Geometry check sheet. Reference: the model listing, model coordinates, mm. A direction names the side the tool comes from. Give positions to 0.01 mm unless a question says otherwise; leave off trailing zeros. Order: outer loops, then holes, each group sorted by start corner. A loop starts at its lowest first (then second) coordinate and runs counter-clockwise, first axis right, second up. Notation, with made-up numbers: M 88,14.5 L 125,14.5 A21 ccw 125,35.5 Z; hole C 5.25,2.5 d4. An arc over 180 degrees is marked long. Answer as CSV lines item,"result".
Autodesk Inventor part; units mm, degrees
ref_plane "YZ Plane" through (0, 0, 0) normal (1, 0, 0) x (0, 1, 0)
ref_plane "XZ Plane" through (0, 0, 0) normal (0, 1, 0) x (-1, 0, 0)
ref_plane "XY Plane" through (0, 0, 0) normal (0, 0, 1) x (1, 0, 0)
sketch "Sketch1" plane through (0, 0, 0) normal (0, 0, 1) x (1, 0, 0)
  line L0 (0, 0) -> (50.8, 0)
  line L1 (50.8, 0) -> (50.8, 5.08)
  line L2 (50.8, 5.08) -> (0, 5.08)
  line L3 (0, 5.08) -> (0, 0)
  line L4 (12.7, 5.08) -> (38.1, 5.08)
  line L5 (38.1, 5.08) -> (38.1, 11.43)
  line L6 (38.1, 11.43) -> (12.7, 11.43)
  line L7 (12.7, 11.43) -> (12.7, 5.08)
  dimension "d0" = 50.8
  dimension "d1" = 5.08
  dimension "d2" = 25.4
  dimension "d3" = 6.35
  dimension "d4" = 12.7
extrude "Extrusion1" add sketch "Sketch1" along normal blind 31.75
sketch "Sketch3" plane through (12.7, 11.43, 0) normal (0, 1, 0) x (1, 0, 0)
  circle A0 centre (12.7, -15.875) radius 3.175
  line L0 (25.4, 0) -> (0, 0)
  line L1 (25.4, 0) -> (25.4, -31.75)
  point P0 (-12.7, 0)
  dimension "d8" = 15.875
  dimension "d9" = 12.7
  dimension "d20" = 6.35
extrude "Extrusion2" cut sketch "Sketch3" against normal blind 2.54
sketch "Sketch4" plane through (0, 5.08, 0) normal (0, 1, 0) x (1, 0, 0)
  circle A0 centre (6.35, -15.875) radius 1.27
  circle A1 centre (44.45, -15.875) radius 1.27
  line L0 (50.8, 0) -> (50.8, -31.75)
  line L1 (0, 0) -> (0, -31.75)
  line L2 (50.8, 0) -> (38.1, 0)
  line L3 (12.7, 0) -> (0, 0)
  dimension "d12" = 2.54
  dimension "d13" = 2.54
  dimension "d14" = 6.35
  dimension "d15" = 6.35
  dimension "d16" = 15.875
  dimension "d17" = 15.875
extrude "Extrusion3" cut sketch "Sketch4" against normal blind 25.4
fillet "Fillet1" radius 0.635 8 edges at (12.7, 11.43, 15.875) (38.1, 11.43, 15.875) (38.1, 5.08, 15.875) (50.8, 5.08, 15.875) (0, 5.08, 15.875) (50.8, 0, 15.875) (0, 0, 15.875) (12.7, 5.08, 15.875)
equation "\"d12\" = d13"
equation "\"d15\" = d14"
equation "\"d17\" = d16"
properties part number "Base"
(1) Material ranges on line 1 (Z direction, x = 6.35, y = 2.5) (3 decimals); line 2 (X direction, y = 8.25, z = 23.5); line 3 (Y direction, x = 47.5, z = 18), recorded low to high.
The answers:
line 1,"z = 0 to 14.605, 17.145 to 31.75"
line 2,"x = 12.7 to 38.1"
line 3,"y = 0 to 5.08"
(2) Section check A-A on x = 44.45. Enter the section's corners in (y, z) (3 decimals).
The answers:
outline,"M 0,0 L 5.08,0 L 5.08,14.605 L 0,14.605 Z; M 0,17.145 L 5.08,17.145 L 5.08,31.75 L 0,31.75 Z"
(3) Section check B-B on x = 25.4. Enter the section's corners in (y, z).
The answers:
outline,"M 0,0 L 11.43,0 L 11.43,12.7 L 8.89,12.7 L 8.89,19.05 L 11.43,19.05 L 11.43,31.75 L 0,31.75 Z"
(4) Section check D-D on x = 4. Enter the section's corners in (y, z).
The answers:
outline,"M 0,0 L 5.08,0 L 5.08,31.75 L 0,31.75 Z"
(5) Tool access check on faces 4 (the face through (50.8, 3, 16)), 5 (the face through (28.43, 10.18, 14.92)), 6 (the face through (46, 5.08, 16)), 7 (the face through (8, 5.08, 16)). Record the directions out of +Z, -Z, +X, -X, +Y, -Y that give a thin tool (end or side, any length) a straight path to the whole face; none if there is none.
The answers:
face 4,"+Z, -Z, +X, +Y, -Y"
face 5,"+Y"
face 6,"+Z, -Z, +X, +Y"
face 7,"+Z, -Z, -X, +Y"
(6) Draft check along X on faces 1 (the face through (25, 8.89, 16)), 2 (the face through (25, 5, 0)), 3 (the face through (38.1, 8, 16)). Enter one of: +X half, -X half, draft (parallel to the pull), parting line (faces both ways), or undercut.
The answers:
face 1,"undercut"
face 2,"draft"
face 3,"+X half"
(7) Gauge pin test, flat ends, axial feed: P1, Ø4, axis at y = 9, z = 11, coming from the -X side; P2, Ø3, axis at x = 25.5, z = 16.5, coming from the +Y side; P3, Ø4, axis at y = 8, z = 18, coming from the +X side. Record the tip position at first contact, or that the pin passes through.
The answers:
P1,"stops at x = 12.7"
P2,"stops at y = 8.89"
P3,"stops at x = 38.1"
(8) Section check C-C on z = 10. Enter the section's corners in (x, y) (3 decimals).
The answers:
outline,"M 0,0.635 A0.635 ccw 0.635,0 L 50.165,0 A0.635 ccw 50.8,0.635 L 50.8,4.445 A0.635 ccw 50.165,5.08 L 38.735,5.08 A0.635 cw 38.1,5.715 L 38.1,10.795 A0.635 ccw 37.465,11.43 L 13.335,11.43 A0.635 ccw 12.7,10.795 L 12.7,5.715 A0.635 cw 12.065,5.08 L 0.635,5.08 A0.635 ccw 0,4.445 Z"
